Could you check a few things on this model? Use its own coordinates, in mm. A direction names the side the tool comes from. Round coordinates to 2 decimals unless told otherwise and drop trailing zeros. Write each loop counter-clockwise with the first axis right and the second up, starting at its lowest first coordinate (ties: lowest second). Pieces come first, ordered by that corner, then holes. Notation, with made-up numbers: (78.5, 25) -> (90.5, 25) arc R19 cw to (90.5, 60) -> close; hole circle Ø3 at (-37, 36.5). An arc over 180 degrees is marked (long way). Answer in a Markdown table with one row per item.
from build123d import *

# Parameters (mm, degrees)
SKETCH1_R           = 31.25
BOSS_EXTRUDE1_DEPTH = 100
BOSS_EXTRUDE2_DEPTH = 30
SKETCH3_W           = 28.564064606
SKETCH3_H           = 90
CUT_EXTRUDE1_DEPTH  = 20


with BuildPart() as part:
    # Sketch1 → Boss-Extrude1 (new body)
    with BuildSketch(Plane.XY):
        Circle(SKETCH1_R)
    extrude(amount=BOSS_EXTRUDE1_DEPTH)

    # Sketch2 → Boss-Extrude2 (add)
    with BuildSketch(Plane(origin=(0, 0, 0), x_dir=(-1, 0, 0), z_dir=(0, 0, -1))):
        Polygon((69.282032303, 0), (34.641016151, 60), (-34.641016151, 60), (-69.282032303, 0), (-34.641016151, -60), (34.641016151, -60), align=None)
    extrude(amount=BOSS_EXTRUDE2_DEPTH)

    # Sketch3 → Cut-Extrude1 (cut)
    with BuildSketch(Plane(origin=(0, 0, -30), x_dir=(-1, 0, 0), z_dir=(0, 0, -1))):
        Rectangle(SKETCH3_W, SKETCH3_H)
    extrude(amount=-CUT_EXTRUDE1_DEPTH, mode=Mode.SUBTRACT)


solid = part.part
1) Please list where these lines run through material, in increasing order: line 1 (Z direction, x = 15, y = -36); line 2 (X direction, y = 3.5, z = -17.5); line 3 (Z direction, x = 8.5, y = 16.5).
Findings:
| item | result |
|---|---|
| line 1 | z = -30 to 0 |
| line 2 | x = -67.26 to -14.28, 14.28 to 67.26 |
| line 3 | z = -10 to 100 |
2) Imagine slicing it at B-B, the plane y = 27. Please give me the cut outline in (x, z), plus the area to 3 significant figures.
Findings:
| item | result |
|---|---|
| outline | (-53.69, -30) -> (-14.28, -30) -> (-14.28, -10) -> (14.28, -10) -> (14.28, -30) -> (53.69, -30) -> (53.69, 0) -> (15.73, 0) -> (15.73, 100) -> (-15.73, 100) -> (-15.73, 0) -> (-53.69, 0) -> close |
| area | 5,800 mm^2 |
3) Thinking about a two-plate mould opening in X: for faces 1 (the face through (0, -45, -20)), 2 (the face through (0, -60, -15)), 3 (the face through (-51.72, -30.42, -14.79)), which applies, +X half, -X half, draft (parallel to the pull), parting line (faces both ways), or undercut?
Findings:
| item | result |
|---|---|
| face 1 | undercut |
| face 2 | draft |
| face 3 | -X half |
4) For pin 1 (8.5 mm diameter, centred on x = -6, y = -1.5, fed in from -Z); pin 2 (22 mm diameter, centred on y = 14, z = -19, fed in from -X); pin 3 (22 mm diameter, centred on y = 21, z = -24.5, fed in from +X), each with a flat end and sliding along its axis, tell me the tip position at first contact or that it passes through.
Findings:
| item | result |
|---|---|
| pin 1 | stops at z = -10 |
| pin 2 | stops at x = -67.55 |
| pin 3 | stops at x = 63.51 |
5) Imagine slicing it at D-D, the plane x = -28.5. Please give me the cut outline in (y, z).
Findings:
| item | result |
|---|---|
| outline | (-60, -30) -> (60, -30) -> (60, 0) -> (12.82, 0) -> (12.82, 100) -> (-12.82, 100) -> (-12.82, 0) -> (-60, 0) -> close |
6) For faces 4 (the face through (-30, 14, 0)), 5 (the face through (0, 0, 100)), 6 (the face through (-14.282, -1, -20)), which set-ups out of +Z, -Z, +X, -X, +Y, -Y let a thin tool reach every point of the face, with its end or its side?
Findings:
| item | result |
|---|---|
| face 4 | +Z |
| face 5 | +Z, +X, -X, +Y, -Y |
| face 6 | -Z |
7) Imagine slicing it at C-C, the plane z = 28. Please give me the cut outline in (x, y), plus the area to 3 significant figures.
Findings:
| item | result |
|---|---|
| outline | circle Ø62.5 at (0, 0) |
| area | 3,070 mm^2 |
8) Imagine slicing it at A-A, the plane x = 0. Please give me the cut outline in (y, z).
Findings:
| item | result |
|---|---|
| outline | (-60, -30) -> (-45, -30) -> (-45, -10) -> (45, -10) -> (45, -30) -> (60, -30) -> (60, 0) -> (31.25, 0) -> (31.25, 100) -> (-31.25, 100) -> (-31.25, 0) -> (-60, 0) -> close |
